For this review, use the dimensioned drawing (mm, ordinates from the lowest corner) and the shaded views. A direction names the side the tool comes from. Give positions to 0.01 mm unless a question says otherwise; leave off trailing zeros. Write each loop counter-clockwise with the first axis right and the second up, starting at its lowest first coordinate (ties: lowest second). Pieces come first, ordered by that corner, then holes.
1) Draft analysis for pull direction X (two halves, no side actions). For the marked faces 4, 5 and 6, state which applies: pulls with the +X half, pulls with the -X half, needs draft (parallel to the pull), parting line crosses it, or undercut.
2) We need section D-D on y = 15. Give the boundary of the cut face in (x, z), and give its area (3 significant figures).
3) We need section A-A on z = 2.5. Give the boundary of the cut face in (x, y).
4) Wall thickness on line 1 along Y through (x, z) = (51.2, 14.5); line 2 along Y through (x, z) = (7, 1.15); line 3 along X through (y, z) = (36, 2.25): over which ranges is each line inside the solid? List them lowest first.
5) We need section C-C on z = 26.25. Give the boundary of the cut face in (x, y), and give its area (3 significant figures).
6) For P1, Ø3.5, axis at y = 32, z = 20, coming from the +X side; P2, Ø1.5, axis at x = 44, y = 34, coming from the -Z side; P3, Ø4, axis at x = 15.5, z = 17, coming from the +Y side, all flat-tipped, find the tip position at first contact; note any pin that passes through.
7) Machinability: for the marked faces 1, 2 and 3, which of the approach directions +Z, -Z, +X, -X, +Y, -Y give a long, thin tool a straight path to every point of the face, cutting with its end or side? Answer none if there is none.
8) We need section B-B on y = 38. Give the boundary of the cut face in (x, z), and give its area (3 significant figures).
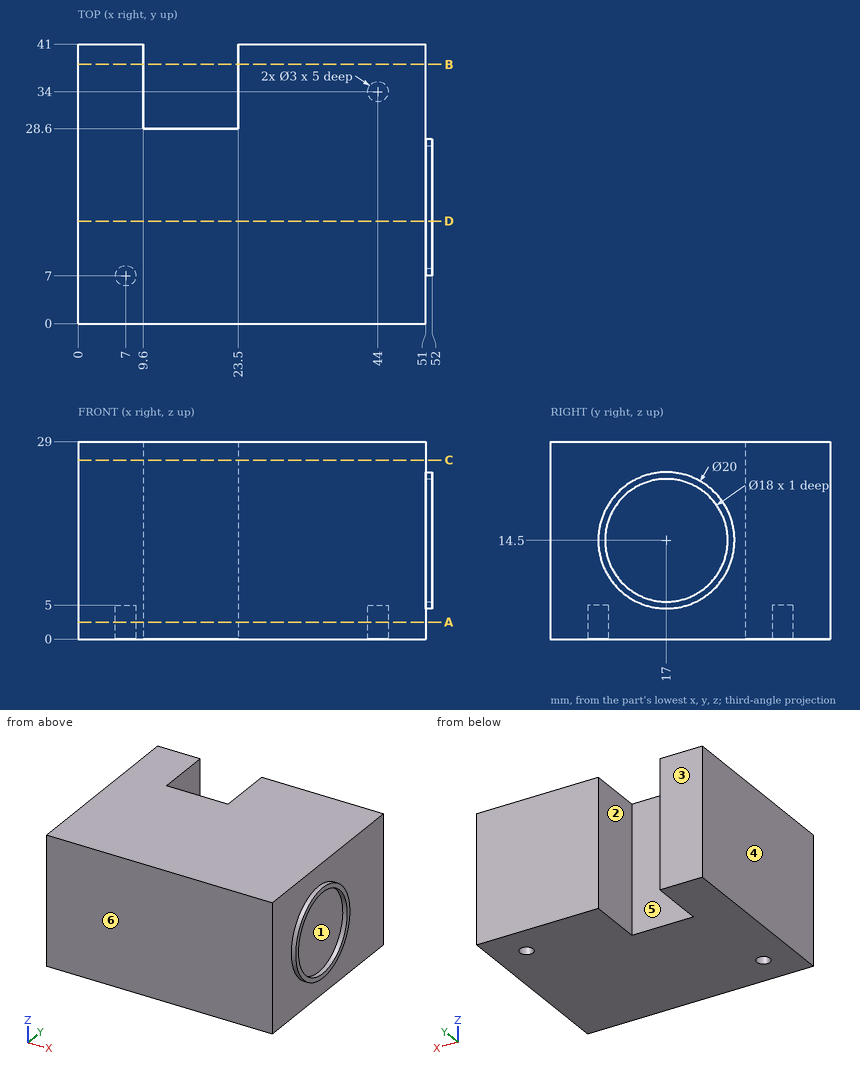
Results list:
1. face 4: pulls with the -X half
1. face 5: undercut
1. face 6: needs draft
2. outline: (0, 0) - (51, 0) - (51, 4.7) - (52, 4.7) - (52, 5.73) - (51, 5.73) - (51, 23.27) - (52, 23.27) - (52, 24.3) - (51, 24.3) - (51, 29) - (0, 29) - close
2. area: 1,480 mm2
3. outline: (0, 0) - (51, 0) - (51, 41) - (23.5, 41) - (23.5, 28.6) - (9.6, 28.6) - (9.6, 41) - (0, 41) - close; hole circle Ø3 at (7, 7); hole circle Ø3 at (44, 34)
4. line 1: y = 7 to 8, 26 to 27
4. line 2: y = 0 to 5.5, 8.5 to 41
4. line 3: x = 0 to 9.6, 23.5 to 51
5. outline: (0, 0) - (51, 0) - (51, 41) - (23.5, 41) - (23.5, 28.6) - (9.6, 28.6) - (9.6, 41) - (0, 41) - close
5. area: 1,920 mm2
6. P1: stops at x = 51
6. P2: stops at z = 5
6. P3: stops at y = 28.6
7. face 1: +X
7. face 2: +Z, -Z, +Y
7. face 3: +Z, -Z, +X, -X, +Y
8. outline: (0, 0) - (9.6, 0) - (9.6, 29) - (0, 29) - close; (23.5, 0) - (51, 0) - (51, 29) - (23.5, 29) - close
8. area: 1,080 mm2
